```python
from build123d import *

# Parameters (mm, degrees)
SKETCH1_W           = 10
SKETCH1_H           = 2.95
BOSS_EXTRUDE1_DEPTH = 2.95
CUT_EXTRUDE1_DEPTH  = 3.95
FILLET1_R           = 11.43
SKETCH3_W           = 2.95
SKETCH3_H           = 10
BOSS_EXTRUDE2_DEPTH = 2.95
SKETCH4_R           = 1.6
CUT_EXTRUDE2_DEPTH  = 3.95


with BuildPart() as part:
    # Sketch1 → Boss-Extrude1 (new body)
    with BuildSketch(Plane.XY):
        Polygon((-2.065, 0), (-12.065, 0), (-12.065, -66.508), (-2.065, -66.508), (17.065, -66.508), (17.065, 0), align=None)
        with Locations((-7.065, 1.475)):
            Rectangle(SKETCH1_W, SKETCH1_H)
        with Locations((-7.065, -67.983)):
            Rectangle(SKETCH1_W, SKETCH1_H)
    extrude(amount=BOSS_EXTRUDE1_DEPTH)

    # Sketch2 → Cut-Extrude1 (cut, through all)
    with BuildSketch(Plane.XY.offset(2.95)):
        Polygon((13.208, -10.773769685), (12.346170522, -10.773769685), (-7.346170522, -55.734230315), (13.208, -55.734230315), align=None)
        Polygon((-7.346170522, -55.734230315), (12.346170522, -10.773769685), (-12.065, -10.773769685), (-12.065, -55.734230315), align=None)
    extrude(amount=-CUT_EXTRUDE1_DEPTH, mode=Mode.SUBTRACT)

    # Fillet1
    fillet1_edges = [part.edges().sort_by_distance(p)[0] for p in [
        (13.208, -10.773769685, 1.475),
        (13.208, -55.734230315, 1.475),
    ]]
    fillet(fillet1_edges, radius=FILLET1_R)

    # Sketch3 → Boss-Extrude2 (add)
    with BuildSketch(Plane.XY.offset(2.95)):
        with BuildLine():
            Line((17.065, -48.254), (17.065, -38.254))
            Line((17.065, -38.254), (17.065, -28.254))
            Line((17.065, -28.254), (17.065, -18.254))
            Line((17.065, -18.254), (12.503866838, -18.254))
            ThreePointArc((12.503866838, -18.254), (13.030589879, -20.197748494), (13.208, -22.203769685))
            Line((13.208, -22.203769685), (13.208, -44.304230315))
            ThreePointArc((13.208, -44.304230315), (13.030589879, -46.310251506), (12.503866838, -48.254))
            Line((12.503866838, -48.254), (17.065, -48.254))
        make_face()
        with Locations((18.54, -23.254)):
            Rectangle(SKETCH3_W, SKETCH3_H)
        with Locations((18.54, -43.254)):
            Rectangle(SKETCH3_W, SKETCH3_H)
    extrude(amount=-BOSS_EXTRUDE2_DEPTH)

    # Sketch4 → Cut-Extrude2 (cut, through all)
    with BuildSketch(Plane.XY.offset(2.95)):
        with Locations((0, -61.508)):
            Circle(SKETCH4_R)
        with Locations((0, -5)):
            Circle(SKETCH4_R)
    extrude(amount=-CUT_EXTRUDE2_DEPTH, mode=Mode.SUBTRACT)


solid = part.part
```
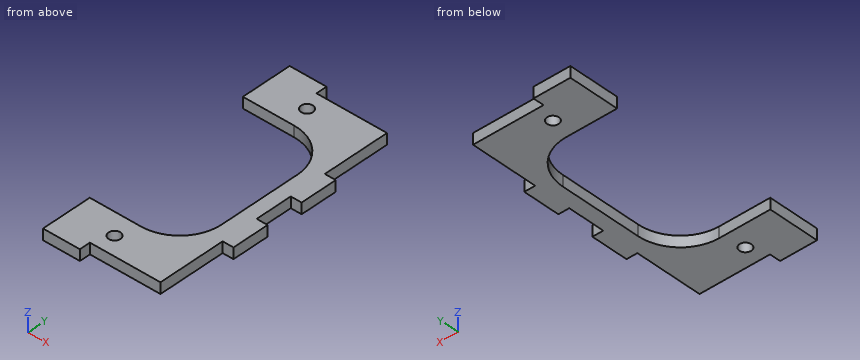
The listing builds one solid part. Answer for the finished solid, in the listing's coordinates (mm). Give positions to 0.01 mm unless a question says otherwise; leave off trailing zeros. Loops run counter-clockwise (first coordinate to the right, second up) from the corner with the lowest first, then second, coordinate; pieces in that order, holes last. Notation, with made-up numbers: (1.5, 77.5) - (24.5, 77.5) arc R22 ccw to (24.5, 93.5) - close; hole circle Ø4 at (63.5, 79). An arc over 180 degrees is marked (long way). Return JSON: item names as keys, results as strings. Group by question number.
1. Find section A-A (y = -5). Write down the section's boundary in (x, z) (3 decimals).
2. Given pin 1 Ø0.9 at (y, z) = (-67.5, 1.5) entering from +X (3 decimals); pin 2 Ø1.5 at (x, z) = (18, 1.5) entering from -Y; pin 3 Ø0.9 at (x, z) = (3.5, 1.5) entering from +Y, each flat-ended and moving along its own axis, determine where each tip first touches the part or whether it passes through.
3. Find section D-D (z = 1.35). Write down the section's boundary in (x, y) (3 decimals).
4. Find section C-C (x = 6). Write down the section's boundary in (y, z), then the cut area to 3 significant figures.
5. Straight lines are drawn through the part: line 1 (Y direction, x = 0, z = 1.05); line 2 (X direction, y = -23, z = 2.6) (3 decimals); line 3 (Y direction, x = 14.5, z = 1.4). For each, find the intervals that lie inside material, in ascending order. Write a range as [from, to].
6. Find section B-B (x = 0). Write down the section's boundary in (y, z).
Verdict:
{
 "1": {"outline": "(-12.065, 0) - (-1.6, 0) - (-1.6, 2.95) - (-12.065, 2.95) - close; (1.6, 0) - (17.065, 0) - (17.065, 2.95) - (1.6, 2.95) - close"},
 "2": {"pin 1": "stops at x = -2.065", "pin 2": "stops at y = -48.25", "pin 3": "stops at y = 0"},
 "3": {"outline": "(-12.065, -69.458) - (-2.065, -69.458) - (-2.065, -66.508) - (17.065, -66.508) - (17.065, -48.254) - (20.015, -48.254) - (20.015, -38.254) - (17.065, -38.254) - (17.065, -28.254) - (20.015, -28.254) - (20.015, -18.254) - (17.065, -18.254) - (17.065, 0) - (-2.065, 0) - (-2.065, 2.95) - (-12.065, 2.95) - (-12.065, -10.774) - (1.778, -10.774) arc R11.43 cw to (13.208, -22.204) - (13.208, -44.304) arc R11.43 cw to (1.778, -55.734) - (-12.065, -55.734) - close; hole circle Ø3.2 at (0, -61.508); hole circle Ø3.2 at (0, -5)"},
 "4": {"outline": "(-66.51, 0) - (-54.93, 0) - (-54.93, 2.95) - (-66.51, 2.95) - close; (-11.58, 0) - (0, 0) - (0, 2.95) - (-11.58, 2.95) - close", "area": "68.3 mm^2"},
 "5": {"line 1": "y = [-66.51, -63.11], [-59.91, -55.73], [-10.77, -6.6], [-3.4, 0]", "line 2": "x = [13.208, 20.015]", "line 3": "y = [-66.51, 0]"},
 "6": {"outline": "(-66.51, 0) - (-63.11, 0) - (-63.11, 2.95) - (-66.51, 2.95) - close; (-59.91, 0) - (-55.73, 0) - (-55.73, 2.95) - (-59.91, 2.95) - close; (-10.77, 0) - (-6.6, 0) - (-6.6, 2.95) - (-10.77, 2.95) - close; (-3.4, 0) - (0, 0) - (0, 2.95) - (-3.4, 2.95) - close"}
}
